Could you check a few things on this model? Use its own coordinates, in mm. Give positions to 0.01 mm unless a question says otherwise; leave off trailing zeros. Order: outer loops, then holes, each group sorted by start corner. A loop starts at its lowest first (then second) coordinate and runs counter-clockwise, first axis right, second up. Notation, with made-up numbers: (82.5, 18.5) -> (131.5, 18.5) arc R13 ccw to (131.5, 30.5) -> close; hole circle Ø5 at (58.5, 2.5). An arc over 180 degrees is marked (long way). Use one line per item in the form item = value. Start each with the question number.
from build123d import *

# Parameters (mm, degrees)
F0_R     = 97.09501
F1_DEPTH = 3


with BuildPart() as f1:
    # F0 (on Front) → F1 (new body)
    with BuildSketch(Plane.XZ):
        with BuildLine():
            Line((-1.5, 115.487013), (-1.5, 122.977865))
            ThreePointArc((-1.5, 122.977865), (-86.964951, 86.964951), (-122.977865, 1.5))
            Line((-122.977865, 1.5), (-115.487013, 1.5))
            Line((-115.487013, 1.5), (-115.487013, -1.5))
            Line((-115.487013, -1.5), (-122.977865, -1.5))
            ThreePointArc((-122.977865, -1.5), (-86.964951, -86.964951), (-1.5, -122.977865))
            Line((-1.5, -122.977865), (-1.5, -115.487013))
            Line((-1.5, -115.487013), (1.5, -115.487013))
            Line((1.5, -115.487013), (1.5, -122.977865))
            ThreePointArc((1.5, -122.977865), (86.964951, -86.964951), (122.977865, -1.5))
            Line((122.977865, -1.5), (115.487013, -1.5))
            Line((115.487013, -1.5), (115.487013, 1.5))
            Line((115.487013, 1.5), (122.977865, 1.5))
            ThreePointArc((122.977865, 1.5), (86.964951, 86.964951), (1.5, 122.977865))
            Line((1.5, 122.977865), (1.5, 115.487013))
            Line((1.5, 115.487013), (-1.5, 115.487013))
        make_face()
        Circle(F0_R, mode=Mode.SUBTRACT)
    extrude(amount=F1_DEPTH)


solid = f1.part
(1) Imagine slicing it at C-C (z = 77). Write out the boundary of the cut face in (x, y).
(2) Imagine slicing it at D-D (z = 105.5). Write out the boundary of the cut face in (x, y), plus the area to 3 significant figures.
(3) Imagine slicing it at B-B (x = -51). Write out the boundary of the cut face in (y, z).
(4) Imagine slicing it at A-A (y = -2.2). Write out the boundary of the cut face in (x, z).
(5) I'm going to push flat-ended pins straight in: pin 1 Ø1.5 at (y, z) = (-2, 0) entering from -X; pin 2 Ø1 at (y, z) = (-1, 80) entering from +X. Where does each tip first touch, or does it pass through?
(6) Please list where these lines run through material, in increasing order: probe 1 along Z at (x, y) = (-0.5, -1.25); probe 2 along X at (y, z) = (-2.7, 45.5); probe 3 along Z at (x, y) = (9.5, -1.7).
Calculated:
q1.outline = (-95.9, -3) -> (-59.15, -3) -> (-59.15, 0) -> (-95.9, 0) -> close; (59.15, -3) -> (95.9, -3) -> (95.9, 0) -> (59.15, 0) -> close
q2.outline = (-63.21, -3) -> (63.21, -3) -> (63.21, 0) -> (-63.21, 0) -> close
q2.area = 379 mm2
q3.outline = (-3, -111.91) -> (0, -111.91) -> (0, -82.62) -> (-3, -82.62) -> close; (-3, 82.62) -> (0, 82.62) -> (0, 111.91) -> (-3, 111.91) -> close
q4.outline = (-122.98, -1.5) arc R122.99 ccw to (-1.5, -122.98) -> (-1.5, -115.49) -> (1.5, -115.49) -> (1.5, -122.98) arc R122.99 ccw to (122.98, -1.5) -> (115.49, -1.5) -> (115.49, 1.5) -> (122.98, 1.5) arc R122.99 ccw to (1.5, 122.98) -> (1.5, 115.49) -> (-1.5, 115.49) -> (-1.5, 122.98) arc R122.99 ccw to (-122.98, 1.5) -> (-115.49, 1.5) -> (-115.49, -1.5) -> close; hole circle Ø194.19 at (0, 0)
q5.pin_1 = -115.49
q5.pin_2 = 93.84
q6.probe_1 = -115.49 to -97.09, 97.09 to 115.49
q6.probe_2 = -114.26 to -85.77, 85.77 to 114.26
q6.probe_3 = -122.62 to -96.63, 96.63 to 122.62
